Build history of the part. All positions in model axes, mm. Face numbers are marked on the shaded views. A direction names the side the tool comes from. Coordinates: 2 decimals unless noted, no trailing zeros. Loops run counter-clockwise (first coordinate to the right, second up) from the corner with the lowest first, then second, coordinate; pieces in that order, holes last. Notation, with made-up numbers: (55, -28.5) -> (71, -28.5) arc R13 ccw to (71, -13.5) -> close; hole circle Ø3 at (38, 17.5). An arc over 180 degrees is marked (long way). One line per item, written item: value. Start each with the question number.
```python
from build123d import *

# Parameters (mm, degrees)
F1_DEPTH       = 2.5
F3_D           = 3.2
F3_CBORE_D     = 6
F3_CBORE_DEPTH = 3.4
F5_D           = 3


with BuildPart() as f1:
    # F0 (on Top) → F1 (new body, symmetric)
    with BuildSketch(Plane.XY):
        Polygon((12, -12.5), (12, 12.5), (8.5, 12.5), (8.5, -0.5), (-8.5, -0.5), (-8.5, 12.5), (-12, 12.5), (-12, -12.5), align=None)
    extrude(amount=F1_DEPTH, both=True)

    # F3 (through all)
    with Locations(Plane.XY.offset(2.5)):
        with Locations((-6.5, -7.5), (6.5, -7.5)):
            CounterBoreHole(F3_D / 2, F3_CBORE_D / 2, F3_CBORE_DEPTH)

    # F5 (through all)
    with Locations(Plane.YZ.offset(12)):
        with Locations((9.5, 0)):
            Hole(F5_D / 2)


solid = f1.part
```
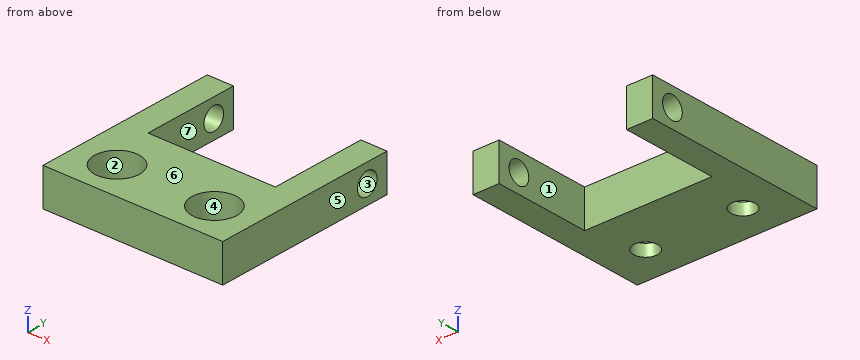
Item 1: Band-saw the part on B-B, the plane y = 6.5. List the corners of the cut face in (x, z).
Item 2: Two-plate mould, pull along X, no slides. Class the marked faces 4, 5, 6 and 7: +X half, -X half, draft (parallel to the pull), parting line (faces both ways), or undercut.
Item 3: Tool access for the marked faces 1, 2 and 3: list every direction of +Z, -Z, +X, -X, +Y, -Y with a clear straight run to the whole face (end or side of a thin tool).
Item 4: Band-saw the part on D-D, the plane x = 6.5. List the corners of the cut face in (y, z), and give its area (3 significant figures).
Item 5: Band-saw the part on C-C, the plane y = 9.5. List the corners of the cut face in (x, z), and give its area (3 significant figures).
Item 6: Band-saw the part on A-A, the plane z = 0. List the corners of the cut face in (x, y).
Item 7: Probe probe 1 along Z at (x, y) = (-9.65, 9.5); probe 2 along Y at (x, z) = (-6.5, 2.2); probe 3 along X at (y, z) = (-6.75, -0.4). List the from-to ranges inside material, lowest first.
Item 8: Drop flat-ended pins along their axis: pin 1 Ø5 at (x, y) = (7.5, -6.5) entering from +Z; pin 2 Ø2.5 at (x, y) = (-6.5, -7.5) entering from -Z. Give the stop position or say it passes through.
Worked out:
1. outline: (-12, -2.5) -> (-8.5, -2.5) -> (-8.5, 2.5) -> (-12, 2.5) -> close; (8.5, -2.5) -> (12, -2.5) -> (12, 2.5) -> (8.5, 2.5) -> close
2. face 4: undercut
2. face 5: +X half
2. face 6: draft
2. face 7: undercut
3. face 1: +Z, -Z, +Y
3. face 2: +Z
3. face 3: +X, -X
4. outline: (-12.5, -2.5) -> (-9.1, -2.5) -> (-9.1, -0.9) -> (-10.5, -0.9) -> (-10.5, 2.5) -> (-12.5, 2.5) -> close; (-5.9, -2.5) -> (-0.5, -2.5) -> (-0.5, 2.5) -> (-4.5, 2.5) -> (-4.5, -0.9) -> (-5.9, -0.9) -> close
4. area: 34.5 mm²
5. outline: (-12, -2.5) -> (-8.5, -2.5) -> (-8.5, -1.5) -> (-12, -1.5) -> close; (-12, 1.5) -> (-8.5, 1.5) -> (-8.5, 2.5) -> (-12, 2.5) -> close; (8.5, -2.5) -> (12, -2.5) -> (12, -1.5) -> (8.5, -1.5) -> close; (8.5, 1.5) -> (12, 1.5) -> (12, 2.5) -> (8.5, 2.5) -> close
5. area: 14.0 mm²
6. outline: (-12, -12.5) -> (12, -12.5) -> (12, 8) -> (8.5, 8) -> (8.5, -0.5) -> (-8.5, -0.5) -> (-8.5, 8) -> (-12, 8) -> close; (-12, 11) -> (-8.5, 11) -> (-8.5, 12.5) -> (-12, 12.5) -> close; (8.5, 11) -> (12, 11) -> (12, 12.5) -> (8.5, 12.5) -> close; hole circle Ø6 at (-6.5, -7.5); hole circle Ø6 at (6.5, -7.5)
7. probe 1: z = -2.5 to -1.5, 1.5 to 2.5
7. probe 2: y = -12.5 to -10.5, -4.5 to -0.5
7. probe 3: x = -12 to -9.4, -3.6 to 3.6, 9.4 to 12
8. pin 1: stops at z = 2.5
8. pin 2: passes through
